Read the model definition and answer for the solid it produces. Units are mm, in the model's axes. Coordinates: 2 decimals unless noted, no trailing zeros. Write each loop counter-clockwise with the first axis right and the second up, starting at its lowest first coordinate (ties: lowest second). Pieces come first, ordered by that corner, then holes. Notation, with made-up numbers: (73, 82) -> (113, 82) arc R34 ccw to (113, 121) -> close; hole circle Ø1 at (-40, 50). An arc over 180 degrees is marked (long way). Answer in a Markdown table with one row per item. Add a question column.
Item 1: Straight lines are drawn through the part: line 1 (Z direction, x = 4, y = 0.3); line 2 (Z direction, x = 11, y = 3.65); line 3 (Z direction, x = 17.5, y = 2.05). For each, find the intervals that lie inside material, in ascending order. Write a range as from..to.
Item 2: Section D-D on x = -20.5 is taken. Write down the section's boundary in (y, z), then the cut area to 3 significant figures.
Item 3: Given pin 1 Ø1 at (y, z) = (3, -19.5) entering from +X; pin 2 Ø1.5 at (y, z) = (1, -37) entering from +X; pin 3 Ø1 at (y, z) = (4, -36) entering from -X; pin 4 Ø3 at (x, z) = (24.71, 4.93) entering from +Y, each flat-ended and moving along its own axis, determine where each tip first touches the part or whether it passes through.
Item 4: Section B-B on x = 0 is taken. Write down the section's boundary in (y, z).
Item 5: Section A-A on z = -8 is taken. Write down the section's boundary in (x, y), then the cut area to 3 significant figures.
Item 6: Section C-C on x = 9.5 is taken. Write down the section's boundary in (y, z).
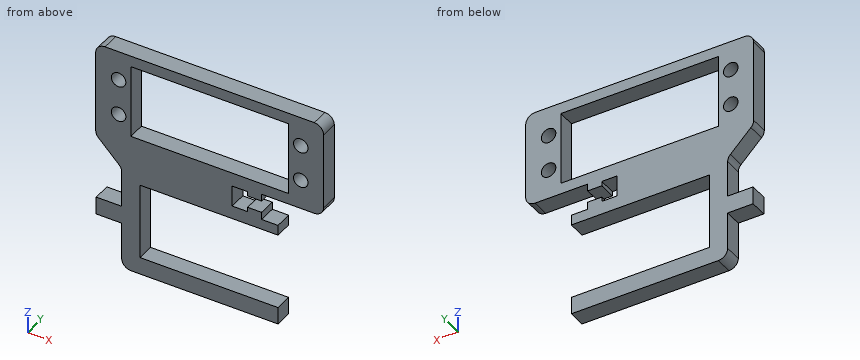
```python
from build123d import *

# Parameters (mm, degrees)
SKETCH1_W               = 42.799
SKETCH1_H               = 19.939
BOSS_EXTRUDE1_DEPTH     = 4.699
FILLET1_R               = 2.54
CUT_EXTRUDE2_DEPTH      = 58.606234053
CUT_EXTRUDE2_DEPTH_BACK = 58.606234053
SKETCH1_3_R             = 1.9685


with BuildPart() as part:
    # Sketch1 → Boss-Extrude1 (new body)
    with BuildSketch(Plane(origin=(0, 0, 0), x_dir=(1, 0, 0), z_dir=(0, 1, 0))):
        Polygon((-23.876, 20.0152), (-30.9245, 12.9667), (-30.9245, -12.9667), (30.9245, -12.9667), (30.9245, 12.9667), (14.097, 12.9667), (14.097, 14.9225), (10.287, 14.9225), (10.287, 13.6779), (6.096, 13.6779), (6.096, 19.3929), (10.287, 19.3929), (10.287, 18.1483), (14.097, 18.1483), (14.097, 20.1803), (18.542, 20.1803), (18.542, 22.9743), (-18.923, 22.9743), (-18.923, 43.6753), (18.542, 43.6753), (18.542, 48.3743), (-23.876, 48.3743), (-23.876, 35.7378), (-30.7848, 35.7378), (-30.7848, 30.9118), (-23.876, 30.9118), align=None)
        Rectangle(SKETCH1_W, SKETCH1_H, mode=Mode.SUBTRACT)
    extrude(amount=BOSS_EXTRUDE1_DEPTH)

    # Fillet1
    fillet1_edges = [part.edges().sort_by_distance(p)[0] for p in [
        (-30.9245, 2.3495, -12.9667),
        (-23.876, 2.3495, -20.0152),
        (-23.876, 2.3495, -48.3743),
        (-30.9245, 2.3495, 12.9667),
        (30.9245, 2.3495, 12.9667),
        (30.9245, 2.3495, -12.9667),
    ]]
    fillet(fillet1_edges, radius=FILLET1_R)

    # Sketch1_3 → Cut-Extrude2 (cut, two sides: drawn at the far end of the back side and taken through both)
    with BuildSketch(Plane(origin=(0, 0, 0), x_dir=(1, 0, 0), z_dir=(0, 1, 0)).offset(-CUT_EXTRUDE2_DEPTH_BACK)):
        with Locations(Location((-24.71166, -4.92506, 0), (0, 0, 270))):
            Circle(SKETCH1_3_R)
        with Locations(Location((24.71166, -4.92506, 0), (0, 0, 270))):
            Circle(SKETCH1_3_R)
        with Locations(Location((24.71166, 4.92506, 0), (0, 0, 270))):
            Circle(SKETCH1_3_R)
        with Locations(Location((-24.71166, 4.92506, 0), (0, 0, 270))):
            Circle(SKETCH1_3_R)
    extrude(amount=CUT_EXTRUDE2_DEPTH + CUT_EXTRUDE2_DEPTH_BACK, mode=Mode.SUBTRACT)


solid = part.part
```
Results below:
| question | item | result |
|---|---|---|
| 1 | line 1 | z = -48.37..-43.68, -22.97..-9.97, 9.97..12.97 |
| 1 | line 2 | z = -48.37..-43.68, -22.97..-18.15, -14.92..-9.97, 9.97..12.97 |
| 1 | line 3 | z = -48.37..-43.68, -22.97..-20.18, -12.97..-9.97, 9.97..12.97 |
| 2 | outline | (0, -48.37) -> (4.7, -48.37) -> (4.7, -9.97) -> (0, -9.97) -> close; (0, 9.97) -> (4.7, 9.97) -> (4.7, 12.97) -> (0, 12.97) -> close |
| 2 | area | 195 mm2 |
| 3 | pin 1 | stops at x = 14.1 |
| 3 | pin 2 | stops at x = -18.92 |
| 3 | pin 3 | stops at x = -30.78 |
| 3 | pin 4 | passes through |
| 4 | outline | (0, -48.37) -> (4.7, -48.37) -> (4.7, -43.68) -> (0, -43.68) -> close; (0, -22.97) -> (4.7, -22.97) -> (4.7, -9.97) -> (0, -9.97) -> close; (0, 9.97) -> (4.7, 9.97) -> (4.7, 12.97) -> (0, 12.97) -> close |
| 5 | outline | (-30.92, 0) -> (-21.4, 0) -> (-21.4, 4.7) -> (-30.92, 4.7) -> close; (21.4, 0) -> (30.92, 0) -> (30.92, 4.7) -> (21.4, 4.7) -> close |
| 5 | area | 89.5 mm2 |
| 6 | outline | (0, -48.37) -> (4.7, -48.37) -> (4.7, -43.68) -> (0, -43.68) -> close; (0, -22.97) -> (4.7, -22.97) -> (4.7, -19.39) -> (0, -19.39) -> close; (0, -13.68) -> (4.7, -13.68) -> (4.7, -9.97) -> (0, -9.97) -> close; (0, 9.97) -> (4.7, 9.97) -> (4.7, 12.97) -> (0, 12.97) -> close |
